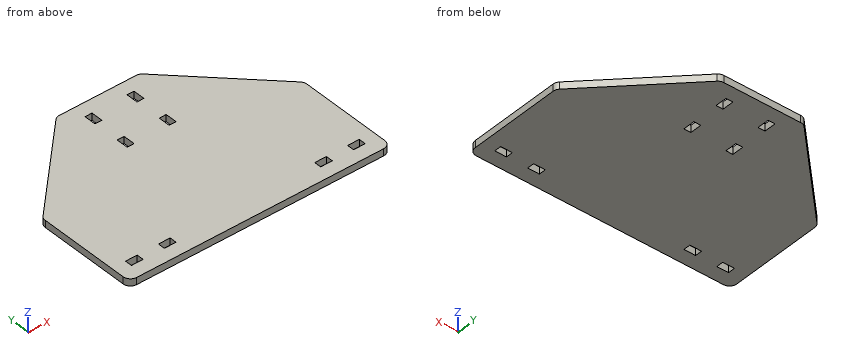
```python
from build123d import *

# Parameters (mm, degrees)
SKETCH1_W           = 8
SKETCH1_H           = 4.7625
SKETCH1_W_2         = 4.7625
SKETCH1_H_2         = 8
BOSS_EXTRUDE1_DEPTH = 4.7625


with BuildPart() as part:
    # Sketch1 → Boss-Extrude1 (new body)
    with BuildSketch(Plane.XY):
        with BuildLine():
            Line((-76.060533906, 57.123033906), (-17.823033906, 115.360533906))
            ThreePointArc((-17.823033906, 115.360533906), (-16.200917162, 116.444397663), (-14.2875, 116.825))
            Line((-14.2875, 116.825), (38.2875, 116.825))
            ThreePointArc((38.2875, 116.825), (40.200917162, 116.444397663), (41.823033906, 115.360533906))
            Line((41.823033906, 115.360533906), (100.060533906, 57.123033906))
            ThreePointArc((100.060533906, 57.123033906), (101.144397663, 55.500917162), (101.525, 53.5875))
            Line((101.525, 53.5875), (101.525, -9.2875))
            ThreePointArc((101.525, -9.2875), (100.060533906, -12.823033906), (96.525, -14.2875))
            Line((96.525, -14.2875), (-72.525, -14.2875))
            ThreePointArc((-72.525, -14.2875), (-76.060533906, -12.823033906), (-77.525, -9.2875))
            Line((-77.525, -9.2875), (-77.525, 53.5875))
            ThreePointArc((-77.525, 53.5875), (-77.144397663, 55.500917162), (-76.060533906, 57.123033906))
        make_face()
        with Locations((-64, -2.38125)):
            Rectangle(SKETCH1_W, SKETCH1_H, mode=Mode.SUBTRACT)
        with Locations((65.481563848, -2.38125)):
            Rectangle(SKETCH1_W, SKETCH1_H, mode=Mode.SUBTRACT)
        with Locations((88, -2.38125)):
            Rectangle(SKETCH1_W, SKETCH1_H, mode=Mode.SUBTRACT)
        with Locations((-2.38125, 77.326723172)):
            Rectangle(SKETCH1_W_2, SKETCH1_H_2, mode=Mode.SUBTRACT)
        with Locations((-2.38125, 103.3)):
            Rectangle(SKETCH1_W_2, SKETCH1_H_2, mode=Mode.SUBTRACT)
        with Locations((26.38125, 77.326723172)):
            Rectangle(SKETCH1_W_2, SKETCH1_H_2, mode=Mode.SUBTRACT)
        with Locations((26.38125, 103.3)):
            Rectangle(SKETCH1_W_2, SKETCH1_H_2, mode=Mode.SUBTRACT)
        with Locations((-41.481563848, -2.38125)):
            Rectangle(SKETCH1_W, SKETCH1_H, mode=Mode.SUBTRACT)
    extrude(amount=BOSS_EXTRUDE1_DEPTH)


solid = part.part
```
Verification items for the finished model (mm, model axes). Give positions to 0.01 mm unless a question says otherwise; leave off trailing zeros. Order: outer loops, then holes, each group sorted by start corner. A loop starts at its lowest first (then second) coordinate and runs counter-clockwise, first axis right, second up. Notation, with made-up numbers: M 76,88.25 L 89,88.25 A18 cw 89,95.25 Z; hole C 66,-20 d6. An arc over 180 degrees is marked long. Answer in a Markdown table with one row per item. Add a question column.
Item 1: Section check C-C, the plane x = -43. Enter the section's corners in (y, z), and give its area (3 significant figures).
Item 2: Scan lines: probe 1 along X at (y, z) = (-0.5, 4.3) (3 decimals); probe 2 along X at (y, z) = (77.5, 0.95); probe 3 along X at (y, z) = (77, 2). Record each from-to range of solid material in increasing order. Write a range as from..to.
Item 3: Gauge pin test, flat ends, axial feed: pin 1 (3 mm diameter, centred on x = -50, y = 72.5, fed in from -Z); pin 2 (1.4 mm diameter, centred on x = 88.5, z = 2, fed in from +Y); pin 3 (1.5 mm diameter, centred on x = -20, z = 4, fed in from +Y); pin 4 (1 mm diameter, centred on x = 77, y = 83.5, fed in from +Z). Record the tip position at first contact, or that the pin passes through.
Item 4: Section check B-B, the plane y = 75.5. Enter the section's corners in (x, z), and give its area (3 significant figures).
Item 5: Section check D-D, the plane z = 1.65. State how many separate pieces and enclosed holes the cut face has, and give its area (3 significant figures).
Item 6: Section check A-A, the plane x = -64. Enter the section's corners in (y, z).
Filled sheet:
| question | item | result |
|---|---|---|
| 1 | outline | M -14.29,0 L -4.76,0 L -4.76,4.76 L -14.29,4.76 Z; M 0,0 L 90.18,0 L 90.18,4.76 L 0,4.76 Z |
| 1 | area | 475 mm^2 |
| 2 | probe 1 | x = -77.525..-68, -60..-45.482, -37.482..61.482, 69.482..84, 92..101.525 |
| 2 | probe 2 | x = -55.68..-4.76, 0..24, 28.76..79.68 |
| 2 | probe 3 | x = -56.18..-4.76, 0..24, 28.76..80.18 |
| 3 | pin 1 | stops at z = 0 |
| 3 | pin 2 | stops at y = 69.38 |
| 3 | pin 3 | stops at y = 113.93 |
| 3 | pin 4 | passes through |
| 4 | outline | M -57.68,0 L -4.76,0 L -4.76,4.76 L -57.68,4.76 Z; M 0,0 L 24,0 L 24,4.76 L 0,4.76 Z; M 28.76,0 L 81.68,0 L 81.68,4.76 L 28.76,4.76 Z |
| 4 | area | 618 mm^2 |
| 5 | separate pieces | 1 |
| 5 | enclosed holes | 8 |
| 5 | area | 19,400 mm^2 |
| 6 | outline | M -14.29,0 L -4.76,0 L -4.76,4.76 L -14.29,4.76 Z; M 0,0 L 69.18,0 L 69.18,4.76 L 0,4.76 Z |
